Here's how the part is built. I have some questions about the finished solid (model axes, mm). A direction names the side the tool comes from. Give positions to 0.01 mm unless a question says otherwise; leave off trailing zeros. Loops run counter-clockwise (first coordinate to the right, second up) from the corner with the lowest first, then second, coordinate; pieces in that order, holes last.
Q1. I'm going to push flat-ended pins straight in: P1, Ø2.5, axis at y = 0, z = 15, coming from the +X side; P2, Ø4, axis at x = 5.5, y = -0.5, coming from the -Z side. Where does each tip first touch, or does it pass through?
Q2. I need wall thicknesses on probe 1 along Z at (x, y) = (8.6, 0); probe 2 along X at (y, z) = (-8.85, 55); probe 3 along X at (y, z) = (2.5, 113). Which ranges of each line are inside material? Lowest first, please.
Q3. Thinking about a two-plate mould opening in X: for faces 1 (the face through (9.01, 0.74, 43.58)), 2 (the face through (0, 8, 74)), 3 (the face through (0.481, 9.014, 56.526)), 4 (the face through (10, 0, 74)), which applies, pulls with the +X half, pulls with the -X half, needs draft (parallel to the pull), parting line crosses it, or undercut?
Q4. Suppose I cut it at C-C (z = 55). List the corners of the cut face in (x, y) for me.
Q5. For faces 5 (the face through (-0.61, -8.99, 6.48)), 6 (the face through (-8, 0, 74)), 7 (the face through (9.014, -0.208, 16.586)), which set-ups out of +Z, -Z, +X, -X, +Y, -Y let a thin tool reach every point of the face, with its end or its side?
Q6. Suppose I cut it at A-A (y = -4.5). List the corners of the cut face in (x, z) for me, and give its area (3 significant figures).
Q7. Suppose I cut it at B-B (x = 0). List the corners of the cut face in (y, z) for me, and give its area (3 significant figures).
```python
from build123d import *

# Parameters (mm, degrees)
SKETCH_1_W          = 20
SKETCH_1_H          = 20
SKETCH_1_W_2        = 16
SKETCH_1_H_2        = 16
EXTRUDE_1_DEPTH     = 150
SKETCH_2_R          = 1.6
CUT_EXTRUDE_1_DEPTH = 408.37168574
SKETCH_3_R          = 1.6
CUT_EXTRUDE_2_DEPTH = 10


with BuildPart() as part:
    # ｽｹｯﾁ1 → ﾎﾞｽ - 押し出し1 (new body)
    with BuildSketch(Plane.XY):
        Rectangle(SKETCH_1_W, SKETCH_1_H)
        Rectangle(SKETCH_1_W_2, SKETCH_1_H_2, mode=Mode.SUBTRACT)
    extrude(amount=EXTRUDE_1_DEPTH)

    # ｽｹｯﾁ2 → ｶｯﾄ - 押し出し1 (cut)
    with BuildSketch(Plane(origin=(0, 10, 0), x_dir=(1, 0, 0), z_dir=(0, 1, 0))):
        with Locations(Location((0, -5, 0), (0, 0, 270))):
            Circle(SKETCH_2_R)
        with Locations(Location((0, -55, 0), (0, 0, 270))):
            Circle(SKETCH_2_R)
    extrude(amount=-CUT_EXTRUDE_1_DEPTH, mode=Mode.SUBTRACT)

    # ｽｹｯﾁ3 → ｶｯﾄ - 押し出し2 (cut)
    with BuildSketch(Plane(origin=(10, 0, 0), x_dir=(0, 0, -1), z_dir=(1, 0, 0))):
        with Locations(Location((-15, 0, 0), (0, 0, 90))):
            Circle(SKETCH_3_R)
        with Locations(Location((-45, 0, 0), (0, 0, 90))):
            Circle(SKETCH_3_R)
    extrude(amount=-CUT_EXTRUDE_2_DEPTH, mode=Mode.SUBTRACT)


solid = part.part
```
Solutions:
1. P1: stops at x = -8
1. P2: passes through
2. probe 1: z = 0 to 13.4, 16.6 to 43.4, 46.6 to 150
2. probe 2: x = -10 to -1.6, 1.6 to 10
2. probe 3: x = -10 to -8, 8 to 10
3. face 1: needs draft
3. face 2: undercut
3. face 3: undercut
3. face 4: pulls with the +X half
4. outline: (-10, -10) - (-1.6, -10) - (-1.6, -8) - (-8, -8) - (-8, 8) - (-1.6, 8) - (-1.6, 10) - (-10, 10) - close; (1.6, -10) - (10, -10) - (10, 10) - (1.6, 10) - (1.6, 8) - (8, 8) - (8, -8) - (1.6, -8) - close
5. face 5: +Y, -Y
5. face 6: +Z, -Z
5. face 7: +X
6. outline: (-10, 0) - (-8, 0) - (-8, 150) - (-10, 150) - close; (8, 0) - (10, 0) - (10, 150) - (8, 150) - close
6. area: 600 mm2
7. outline: (-10, 0) - (-8, 0) - (-8, 3.4) - (-10, 3.4) - close; (-10, 6.6) - (-8, 6.6) - (-8, 53.4) - (-10, 53.4) - close; (-10, 56.6) - (-8, 56.6) - (-8, 150) - (-10, 150) - close; (8, 0) - (10, 0) - (10, 3.4) - (8, 3.4) - close; (8, 6.6) - (10, 6.6) - (10, 53.4) - (8, 53.4) - close; (8, 56.6) - (10, 56.6) - (10, 150) - (8, 150) - close
7. area: 574 mm2
